Could you check a few things on this model? Use its own coordinates, in mm. A direction names the side the tool comes from. Give positions to 0.01 mm unless a question says otherwise; leave off trailing zeros. Write each loop counter-clockwise with the first axis right and the second up, starting at its lowest first coordinate (ties: lowest second). Pieces come first, ordered by that corner, then holes. Notation, with made-up numbers: M 31,-25.75 L 57,-25.75 A19 ccw 57,0.25 Z; hole C 46,-36.5 d1. An arc over 180 degrees is marked long. Answer as a JSON object with one key per item and string values. Group by question number.
```python
from build123d import *

# Parameters (mm, degrees)
SKETCH1_W                        = 86.36
SKETCH1_H                        = 38.1
BOSS_EXTRUDE1_DEPTH              = 3.81
SKETCH2_W                        = 3.81
SKETCH2_H                        = 38.1
BOSS_EXTRUDE2_DEPTH              = 31.75
SKETCH3_W                        = 3.81
SKETCH3_H                        = 38.1
BOSS_EXTRUDE3_DEPTH              = 31.75
SKETCH4_W                        = 3.81
SKETCH4_H                        = 38.1
BOSS_EXTRUDE4_DEPTH              = 3.175
FILLET1_R                        = 1.27
F_10_CLEARANCE_HOLE1_D           = 5.1054
F_10_CLEARANCE_HOLE1_CSINK_D     = 6.3754
F_10_CLEARANCE_HOLE1_CSINK_ANGLE = 90


with BuildPart() as part:
    # Sketch1 → Boss-Extrude1 (new body)
    with BuildSketch(Plane.XY):
        with Locations((-43.18, 19.05)):
            Rectangle(SKETCH1_W, SKETCH1_H)
    extrude(amount=BOSS_EXTRUDE1_DEPTH)

    # Sketch2 → Boss-Extrude2 (add)
    with BuildSketch(Plane.XY.offset(3.81)):
        with Locations((-59.055, 19.05)):
            Rectangle(SKETCH2_W, SKETCH2_H)
    extrude(amount=BOSS_EXTRUDE2_DEPTH)

    # Sketch3 → Boss-Extrude3 (add)
    with BuildSketch(Plane(origin=(-57.15, 0, 0), x_dir=(0, 0, -1), z_dir=(1, 0, 0))):
        with Locations((-33.655, 19.05)):
            Rectangle(SKETCH3_W, SKETCH3_H)
    extrude(amount=BOSS_EXTRUDE3_DEPTH)

    # Sketch4 → Boss-Extrude4 (add)
    with BuildSketch(Plane(origin=(0, 0, 31.75), x_dir=(-1, 0, 0), z_dir=(0, 0, -1))):
        with Locations((27.305, 19.05)):
            Rectangle(SKETCH4_W, SKETCH4_H)
    extrude(amount=BOSS_EXTRUDE4_DEPTH)

    # Fillet1
    fillet1_edges = [part.edges().sort_by_distance(p)[0] for p in [
        (-86.36, 19.05, 3.81),
        (-73.66, 38.1, 3.81),
        (-28.575, 0, 3.81),
        (-57.15, 19.05, 3.81),
        (-60.96, 19.05, 3.81),
        (-73.66, 0, 3.81),
        (-60.96, 38.1, 19.685),
        (-60.96, 0, 19.685),
        (-43.18, 38.1, 35.56),
        (-60.96, 19.05, 35.56),
        (-43.18, 0, 35.56),
        (-57.15, 38.1, 17.78),
        (-57.15, 0, 17.78),
        (-57.15, 19.05, 31.75),
        (-25.4, 19.05, 35.56),
        (-43.18, 38.1, 31.75),
        (-43.18, 0, 31.75),
        (-25.4, 19.05, 28.575),
        (-27.305, 0, 28.575),
        (-29.21, 19.05, 28.575),
        (-27.305, 38.1, 28.575),
        (0, 19.05, 3.81),
        (0, 0, 1.905),
        (-86.36, 0, 1.905),
        (-86.36, 38.1, 1.905),
        (0, 38.1, 1.905),
        (-28.575, 38.1, 3.81),
    ]]
    fillet(fillet1_edges, radius=FILLET1_R)

    # #10 Clearance Hole1 (through all)
    with Locations(Plane.XY.offset(3.81)):
        with Locations((-73.66, 11.43), (-73.66, 26.67), (-12.7, 11.43), (-12.7, 26.67)):
            CounterSinkHole(F_10_CLEARANCE_HOLE1_D / 2, F_10_CLEARANCE_HOLE1_CSINK_D / 2, counter_sink_angle=F_10_CLEARANCE_HOLE1_CSINK_ANGLE)


solid = part.part
```
1) For faces 5 (the flat face through (-86.36, 19, 1)), 6 (the flat face through (0, 19, 1)), 7 (the flat face through (-25.4, 19, 32)), 8 (the flat face through (-43, 19, 31.75)), 9 (the flat face through (-60.96, 19, 19)), which set-ups out of +Z, -Z, +X, -X, +Y, -Y let a thin tool reach every point of the face, with its end or its side?
2) We'd pull the mould along Z, two halves only. Please class faces 1 (the cylindrical face through (-15.058, 10.452, 1.565)), 2 (the flat face through (-29, 19, 3.81)), 3 (the flat face through (-57.15, 19, 18)), 4 (the flat face through (-74, 19, 3.81)): released by +Z, released by -Z, zero draft, split by the parting line, or undercut.
3) If we section it at C-C, the plane x = -73.66: List the corners of the cut face in (y, z) for me (3 decimals).
4) If we section it at A-A, the plane x = -34: List the corners of the cut face in (y, z) for me, plus the area to 3 significant figures.
5) If we section it at B-B, the plane y = 11.43: Give the number of separate pieces and of enclosed holes in the cut face, plus the area to 3 significant figures.
6) Please list where these lines run through material, in increasing order: line 1 along X through (y, z) = (26.67, 0.8); line 2 along Y through (x, z) = (-73.66, 2.3); line 3 along Z through (x, y) = (-46, 33.5). Write a range as from..to.
7) If we section it at D-D, the plane z = 24.5: List the corners of the cut face in (x, y) for me, plus the area to 3 significant figures.
8) I'm going to push flat-ended pins straight in: pin 1 (1 mm diameter, centred on x = -39, y = 5.5, fed in from -Z); pin 2 (4 mm diameter, centred on x = -12.7, y = 26.67, fed in from +Z); pin 3 (2 mm diameter, centred on y = 27, z = 32.5, fed in from +X); pin 4 (7.5 mm diameter, centred on y = 20.5, z = 20.5, fed in from +X). Where does each tip first touch, or does it pass through?
Taken from the geometry:
{
 "1": {"face 5": "+Z, -Z, -X, +Y, -Y", "face 6": "+Z, -Z, +X, +Y, -Y", "face 7": "+Z, +X, +Y, -Y", "face 8": "+Y, -Y", "face 9": "+Z, -X, +Y, -Y"},
 "2": {"face 1": "zero draft", "face 2": "undercut", "face 3": "undercut", "face 4": "released by +Z"},
 "3": {"outline": "M 0,0 L 8.877,0 L 8.877,3.175 L 8.242,3.81 L 1.27,3.81 A1.27 ccw 0,2.54 Z; M 13.983,0 L 24.117,0 L 24.117,3.175 L 23.482,3.81 L 14.618,3.81 L 13.983,3.175 Z; M 29.223,0 L 38.1,0 L 38.1,2.54 A1.27 ccw 36.83,3.81 L 29.858,3.81 L 29.223,3.175 Z"},
 "4": {"outline": "M 0,0 L 38.1,0 L 38.1,2.54 A1.27 ccw 36.83,3.81 L 1.27,3.81 A1.27 ccw 0,2.54 Z; M 0,33.02 A1.27 ccw 1.27,31.75 L 36.83,31.75 A1.27 ccw 38.1,33.02 L 38.1,34.29 A1.27 ccw 36.83,35.56 L 1.27,35.56 A1.27 ccw 0,34.29 Z", "area": "288 mm²"},
 "5": {"separate pieces": "3", "enclosed holes": "0", "area": "542 mm²"},
 "6": {"line 1": "-86.36..-76.21, -71.11..-15.25, -10.15..0", "line 2": "0..8.88, 13.98..24.12, 29.22..38.1", "line 3": "0..3.81, 31.75..35.56"},
 "7": {"outline": "M -60.96,1.27 A1.27 ccw -59.69,0 L -58.42,0 A1.27 ccw -57.15,1.27 L -57.15,36.83 A1.27 ccw -58.42,38.1 L -59.69,38.1 A1.27 ccw -60.96,36.83 Z", "area": "144 mm²"},
 "8": {"pin 1": "z = 0", "pin 2": "through", "pin 3": "x = -25.4", "pin 4": "x = -57.15"}
}
